```python
from build123d import *

# Parameters (mm, degrees)
F1_DEPTH  = 40
F3_DEPTH  = 70.001
F4_R      = 2.5
F5_DEPTH  = 1
F6_R      = 2.5
F7_DEPTH  = 1
F8_R      = 2.5
F9_DEPTH  = 1
F10_R     = 2.5
F11_DEPTH = 1
F13_DEPTH = 1
F15_DEPTH = 1
F17_DEPTH = 1
F19_DEPTH = 1


with BuildPart() as f1:
    # F0 (on Front) → F1 (new body)
    with BuildSketch(Plane.XZ):
        with BuildLine():
            Line((-35, -5), (35, -5))
            Line((35, -5), (35, 5))
            Line((35, 5), (27.5, 5))
            ThreePointArc((27.5, 5), (20, -2.5), (12.5, 5))
            Line((12.5, 5), (7.5, 5))
            ThreePointArc((7.5, 5), (0, -2.5), (-7.5, 5))
            Line((-7.5, 5), (-12.5, 5))
            ThreePointArc((-12.5, 5), (-20, -2.5), (-27.5, 5))
            Line((-27.5, 5), (-35, 5))
            Line((-35, 5), (-35, -5))
        make_face()
    extrude(amount=F1_DEPTH)

    # F2 (on face) → F3 (cut, through all)
    with BuildSketch(Plane.YZ.offset(35)):
        with BuildLine():
            ThreePointArc((-27.5, 5), (-20, -2.5), (-12.5, 5))
            Line((-12.5, 5), (-27.5, 5))
        make_face()
    extrude(amount=-F3_DEPTH, mode=Mode.SUBTRACT)

    # F4 (on face) → F5 (cut)
    with BuildSketch(Plane.XY.offset(5)):
        with Locations((31, -36)):
            Circle(F4_R)
    extrude(amount=-F5_DEPTH, mode=Mode.SUBTRACT)

    # F6 (on face) → F7 (cut)
    with BuildSketch(Plane.XY.offset(5)):
        with Locations((31, -3.9921798557)):
            Circle(F6_R)
    extrude(amount=-F7_DEPTH, mode=Mode.SUBTRACT)

    # F8 (on face) → F9 (cut)
    with BuildSketch(Plane.XY.offset(5)):
        with Locations((-31, -36)):
            Circle(F8_R)
    extrude(amount=-F9_DEPTH, mode=Mode.SUBTRACT)

    # F10 (on face) → F11 (cut)
    with BuildSketch(Plane.XY.offset(5)):
        with Locations((-31, -4)):
            Circle(F10_R)
    extrude(amount=-F11_DEPTH, mode=Mode.SUBTRACT)

    # F12 (on face) → F13 (cut)
    with BuildSketch(Plane.XY.offset(5)):
        with BuildLine():
            ThreePointArc((-12.5, -4), (-10, -6.5), (-7.5, -4))
            ThreePointArc((-7.5, -4), (-10, -1.5), (-12.5, -4))
        make_face()
    extrude(amount=-F13_DEPTH, mode=Mode.SUBTRACT)

    # F14 (on face) → F15 (cut)
    with BuildSketch(Plane.XY.offset(5)):
        with BuildLine():
            ThreePointArc((7.5, -4), (10, -6.5), (12.5, -4))
            ThreePointArc((12.5, -4), (10, -1.5), (7.5, -4))
        make_face()
    extrude(amount=-F15_DEPTH, mode=Mode.SUBTRACT)

    # F16 (on face) → F17 (cut)
    with BuildSketch(Plane.XY.offset(5)):
        with BuildLine():
            ThreePointArc((-12.5, -36), (-10, -38.5), (-7.5, -36))
            ThreePointArc((-7.5, -36), (-10, -33.5), (-12.5, -36))
        make_face()
    extrude(amount=-F17_DEPTH, mode=Mode.SUBTRACT)

    # F18 (on face) → F19 (cut)
    with BuildSketch(Plane.XY.offset(5)):
        with BuildLine():
            ThreePointArc((7.5, -36), (10, -38.5), (12.5, -36))
            ThreePointArc((12.5, -36), (10, -33.5), (7.5, -36))
        make_face()
    extrude(amount=-F19_DEPTH, mode=Mode.SUBTRACT)


solid = f1.part
```
Can you work these out from the model? Positions are in its coordinate system, mm. A direction names the side the tool comes from. Coordinates: 2 decimals unless noted, no trailing zeros. Write each loop counter-clockwise with the first axis right and the second up, starting at its lowest first coordinate (ties: lowest second). Pieces come first, ordered by that corner, then holes. Notation, with made-up numbers: M 50,-4 L 56,-4 A21 ccw 56,6 Z; hole C 61.25,2 d4. An arc over 180 degrees is marked long. Write item = value, one per line. Start each with the question number.
Q1. If I drill on L1, parallel to Y at x = 31, z = 4.55; L2, parallel to X at y = -30, z = 3.5; L3, parallel to X at y = -32, z = 4, over which ranges is the centre line in solid material (lowest first)? Write a range as [from, to].
Q2. Thinking about a two-plate mould opening in X: for faces 3 (the face through (35, -20, -3)), 4 (the face through (-9.86, -20.16, -2.5)), 5 (the face through (0.16, -7.64, -2.5)), which applies, released by +X, released by -X, zero draft, split by the parting line, or undercut?
Q3. If we section it at C-C, the plane x = -31: Write out the boundary of the cut face in (y, z), then the cut area to 3 significant figures.
Q4. If we section it at A-A, the plane z = 2: State how many separate pieces and enclosed holes the cut face has, then the cut area to 3 significant figures.
Q5. On a 3-axis mill with a long thin cutter (end or side, diameter ignored), from which of +Z, -Z, +X, -X, +Y, -Y can I reach the whole of each face in a straight line? I mean faces 1 (the face through (0.16, -32.08, -2.5)), 2 (the face through (-10, -36, 4)). Say none if no direction works.
Q6. I'm going to push flat-ended pins straight in: pin 1 (5 mm diameter, centred on x = -1, y = -6.5, fed in from +Z); pin 2 (2.5 mm diameter, centred on x = 10, y = -5, fed in from +Z); pin 3 (2 mm diameter, centred on x = -1, y = -20, fed in from +Z). Where does each tip first touch, or does it pass through?
Q7. If we section it at D-D, the plane y = -37: Write out the boundary of the cut face in (x, z).
Q8. If we section it at B-B, the plane y = -9: Write out the boundary of the cut face in (x, z), then the cut area to 3 significant figures.
Check sheet entries:
q1.L1 = [-40, -38.5], [-33.5, -27.49], [-12.51, -6.49], [-1.49, 0]
q1.L2 = [-35, -27.35], [-12.65, -7.35], [7.35, 12.65], [27.35, 35]
q1.L3 = [-35, -27.43], [-12.57, -7.43], [7.43, 12.57], [27.43, 35]
q2.face_3 = released by +X
q2.face_4 = zero draft
q2.face_5 = undercut
q3.outline = M -40,-5 L 0,-5 L 0,5 L -1.5,5 L -1.5,4 L -6.5,4 L -6.5,5 L -12.5,5 A7.5 cw -27.5,5 L -33.5,5 L -33.5,4 L -38.5,4 L -38.5,5 L -40,5 Z
q3.area = 302 mm²
q4.separate_pieces = 8
q4.enclosed_holes = 0
q4.area = 755 mm²
q5.face_1 = +Z, +Y, -Y
q5.face_2 = +Z
q6.pin_1 = -1.63
q6.pin_2 = 4
q6.pin_3 = -2.43
q7.outline = M -35,-5 L 35,-5 L 35,5 L 33.29,5 L 33.29,4 L 28.71,4 L 28.71,5 L 27.5,5 A7.5 cw 12.5,5 L 12.29,5 L 12.29,4 L 7.71,4 L 7.71,5 L 7.5,5 A7.5 cw -7.5,5 L -7.71,5 L -7.71,4 L -12.29,4 L -12.29,5 L -12.5,5 A7.5 cw -27.5,5 L -28.71,5 L -28.71,4 L -33.29,4 L -33.29,5 L -35,5 Z
q8.outline = M -35,-5 L 35,-5 L 35,5 L 27.5,5 A7.5 cw 12.5,5 L 7.5,5 A7.5 cw -7.5,5 L -12.5,5 A7.5 cw -27.5,5 L -35,5 Z
q8.area = 435 mm²
